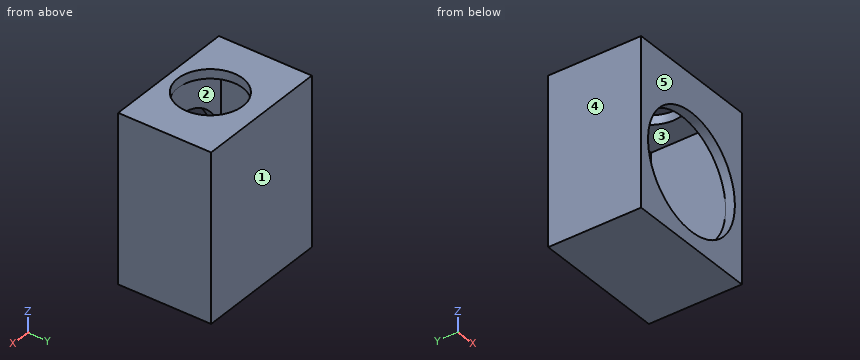
Autodesk Inventor part; units mm, degrees
ref_plane "YZ Plane" through (0, 0, 0) normal (1, 0, 0) x (0, 1, 0)
ref_plane "XZ Plane" through (0, 0, 0) normal (0, 1, 0) x (-1, 0, 0)
ref_plane "XY Plane" through (0, 0, 0) normal (0, 0, 1) x (1, 0, 0)
sketch "Sketch1" plane through (0, 0, 0) normal (0, 1, 0) x (-1, 0, 0)
  line L0 (-7.25, -9) -> (7.25, -9)
  line L1 (7.25, -9) -> (7.25, 9)
  line L2 (7.25, 9) -> (-7.25, 9)
  line L3 (-7.25, 9) -> (-7.25, -9)
  line L4 (-7.25, -9) -> (7.25, 9) construction
  line L5 (7.25, -9) -> (-7.25, 9) construction
  point P0 (0, 0)
  dimension "d0" = 14.5
  dimension "d1" = 18
extrude "Extrusion1" add sketch "Sketch1" along normal blind 8 and the other way blind 1
sketch "Sketch2" plane through (0, -1, 0) normal (0, -1, 0) x (1, 0, 0)
  line L0 (-7.25, 9) -> (-7.25, -9)
  line L1 (-7.25, -9) -> (7.25, -9)
  circle A0 centre (0, -1.25) radius 6.25
  point P0 (0, 0)
  dimension "d7" = 1.5
  dimension "d8" = 1
  dimension "d9" = 12.5
extrude "Extrusion2" cut sketch "Sketch2" against normal blind 8
sketch "Sketch3" plane through (-7.25, 8, 9) normal (0, 0, 1) x (1, 0, 0)
  line L0 (0, 0) -> (14.5, 0)
  circle A0 centre (7.25, -4.5) radius 3.5
  point P0 (7.25, -8)
  dimension "d14" = 1
extrude "Extrusion3" cut sketch "Sketch3" against normal blind 8
sketch "Sketch4" plane through (0, 8, 0) normal (0, 1, 0) x (1, 0, 0)
  line L0 (-7.25, 9) -> (-7.25, -9)
  line L1 (-7.25, -9) -> (7.25, -9)
  line L2 (7.25, -9) -> (7.25, 9)
  line L3 (7.25, 9) -> (-7.25, 9)
  line L4 (6.25, -8) -> (-6.25, -8)
  line L5 (-6.25, -8) -> (-6.25, 8)
  line L6 (-6.25, 8) -> (6.25, 8)
  line L7 (6.25, 8) -> (6.25, -8)
  point P0 (0, 0)
  dimension "d17" = 1
  dimension "d18" = 1
  dimension "d19" = 1
  dimension "d20" = 1
extrude "Extrusion4" cut sketch "Sketch4" against normal blind 8 contours L4 L5 L6 L7
sketch "Sketch5" plane through (0, 8, 0) normal (0, 1, 0) x (1, 0, 0)
  line L0 (-7.25, 9) -> (-7.25, -9)
  line L1 (-7.25, -9) -> (7.25, -9)
  line L2 (7.25, -9) -> (7.25, 9)
  line L3 (7.25, 9) -> (-7.25, 9)
  line L4 (7.25, -9) -> (-7.25, -9)
  line L5 (7.25, 9) -> (-7.25, 9)
  line L6 (-7.25, 9) -> (-7.25, -9)
  line L7 (-7.25, -9) -> (7.25, -9)
  line L8 (7.25, -9) -> (7.25, 9)
  point P0 (0, 0)
extrude "Extrusion5" add sketch "Sketch5" along normal blind 1
properties part number "carcasaXeotype_BUZZER"
The listing builds one solid part. Answer for the finished solid, in the listing's coordinates (mm). Face numbers are marked on the shaded views. A direction names the side the tool comes from. Give positions to 0.01 mm unless a question says otherwise; leave off trailing zeros. Write each loop counter-clockwise with the first axis right and the second up, starting at its lowest first coordinate (ties: lowest second). Pieces come first, ordered by that corner, then holes. Notation, with made-up numbers: (69.5, -11) -> (94.5, -11) arc R6 cw to (94.5, -2) -> close; hole circle Ø5 at (-26, 89). An arc over 180 degrees is marked (long way). One line per question, with ' | ' between items. Start each with the question number.
1. Section C-C (z = -5.75) is taken. Determine the outline of the cut face in (x, y), plus the area to 3 significant figures.
2. Find the intervals of material crossed by probe 1 along X at (y, z) = (7.75, -3.5); probe 2 along Z at (x, y) = (-4.5, 3.5); probe 3 along Y at (x, z) = (5.25, 6.75), in increasing order.
3. Section A-A (y = 3.5) is taken. Determine the outline of the cut face in (x, z).
4. For a pull along Y with two mould halves and no side action, classify the marked faces 3, 4 and 5 as pulls with the +Y half, pulls with the -Y half, needs draft (parallel to the pull), parting line crosses it, or undercut.
5. Given pin 1 Ø1.5 at (x, y) = (-0.5, 6) entering from +Z; pin 2 Ø2 at (x, z) = (2.5, 0.5) entering from -Y, each flat-ended and moving along its own axis, determine where each tip first touches the part or whether it passes through.
6. For the marked faces 1 and 2, determine the directions among +Z, -Z, +X, -X, +Y, -Y from which every point of the face is accessible in a straight line to the end or side of a thin tool.
7. Section B-B (x = -1.75) is taken. Determine the outline of the cut face in (y, z).
Response values:
1) outline: (-7.25, -1) -> (-4.34, -1) -> (-4.34, 0) -> (-6.25, 0) -> (-6.25, 8) -> (6.25, 8) -> (6.25, 0) -> (4.34, 0) -> (4.34, -1) -> (7.25, -1) -> (7.25, 9) -> (-7.25, 9) -> close | area: 36.3 mm2
2) probe 1: -7.25 to -6.25, 6.25 to 7.25 | probe 2: -9 to -8, 8 to 9 | probe 3: -1 to 0, 8 to 9
3) outline: (-7.25, -9) -> (7.25, -9) -> (7.25, 9) -> (3.5, 9) -> (3.5, 8) -> (6.25, 8) -> (6.25, -8) -> (-6.25, -8) -> (-6.25, 8) -> (-3.5, 8) -> (-3.5, 9) -> (-7.25, 9) -> close
4) face 3: undercut | face 4: needs draft | face 5: pulls with the -Y half
5) pin 1: z = -8 | pin 2: y = 8
6) face 1: +Z, -Z, +X, -X, +Y | face 2: none
7) outline: (-1, -9) -> (9, -9) -> (9, 9) -> (6.53, 9) -> (6.53, 8) -> (8, 8) -> (8, -8) -> (0, -8) -> (0, -7.25) -> (-1, -7.25) -> close; (-1, 4.75) -> (0, 4.75) -> (0, 8) -> (0.47, 8) -> (0.47, 9) -> (-1, 9) -> close
